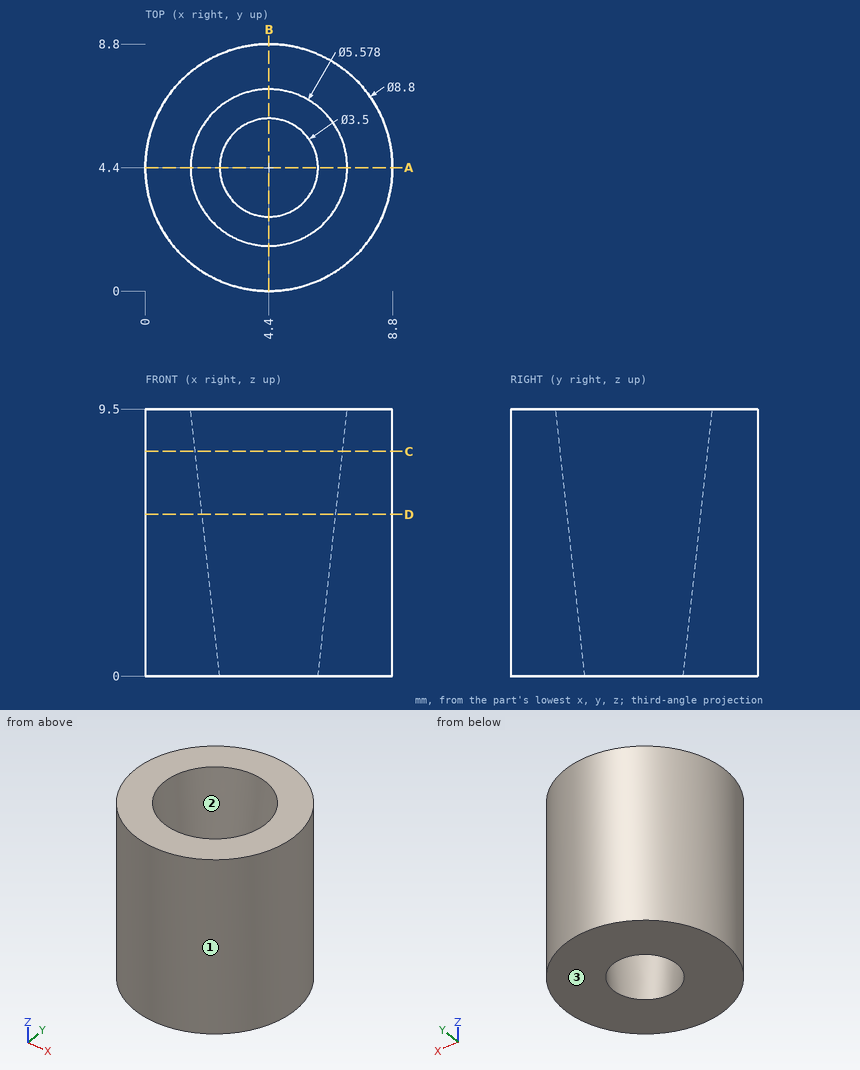
Drawing for the job (mm, zero at the part's lowest x, y, z). Round coordinates to 2 decimals unless told otherwise and drop trailing zeros. Order: outer loops, then holes, each group sorted by start corner. A loop starts at its lowest first (then second) coordinate and runs counter-clockwise, first axis right, second up.
Item 1: Mould opens along X. For the marked faces 1, 2 and 3 say: pulls with the +X half, pulls with the -X half, needs draft (parallel to the pull), parting line crosses it, or undercut.
Item 2: Saw through at C-C on z = 8. Write the cut outline in (x, y) (3 decimals).
Item 3: Pin check, flat tip, straight feed: pin 1 (3 mm diameter, centred on y = 2.5, z = 7, fed in from +X). Stop position of the tip, or through.
Item 4: Probe line 1 along Y through (x, z) = (2.5, 8); line 2 along Y through (x, z) = (5, 1.5); line 3 along X through (y, z) = (4.25, 2). List the from-to ranges inside material, lowest first.
Item 5: Saw through at D-D on z = 5.75. Write the cut outline in (x, y).
Item 6: Saw through at A-A on y = 4.4. Write the cut outline in (x, z), then the cut area to 3 significant figures.
Reported:
1. face 1: parting line crosses it
1. face 2: undercut
1. face 3: needs draft
2. outline: circle Ø8.8 at (4.4, 4.4); hole circle Ø5.25 at (4.4, 4.4)
3. pin 1: stops at x = 8.78
4. line 1: y = 0.43 to 2.59, 6.21 to 8.37
4. line 2: y = 0.04 to 2.58, 6.22 to 8.76
4. line 3: x = 0 to 2.44, 6.36 to 8.8
5. outline: circle Ø8.8 at (4.4, 4.4); hole circle Ø4.76 at (4.4, 4.4)
6. outline: (0, 0) - (2.65, 0) - (1.61, 9.5) - (0, 9.5) - close; (6.15, 0) - (8.8, 0) - (8.8, 9.5) - (7.19, 9.5) - close
6. area: 40.5 mm2
